Could you check a few things on this model? Use its own coordinates, in mm. A direction names the side the tool comes from. Round coordinates to 2 decimals unless told otherwise and drop trailing zeros. Write each loop counter-clockwise with the first axis right and the second up, starting at its lowest first coordinate (ties: lowest second). Pieces come first, ordered by that corner, then holes. Notation, with made-up numbers: (33, 73.5) -> (83, 73.5) arc R25 ccw to (83, 95.5) -> close; hole circle Ø4 at (-31, 27.5). An arc over 180 degrees is marked (long way). One line per question, with ' | ' between items. Start each with the question number.
1. Thinking about a two-plate mould opening in X: for faces 4 (the flat face through (12.7, 1.5, -4.1)), 5 (the flat face through (7, 0.8, -4)), 6 (the flat face through (9.064, 2.803, -3.514)), 7 (the flat face through (6, -1, -8)), which applies, released by +X, released by -X, zero draft, split by the parting line, or undercut?
2. Imagine slicing it at B-B, the plane z = -1. List the corners of the cut face in (x, y) for me.
3. If I drill on line 1 along Y through (x, z) = (11.5, -1); line 2 along Y through (x, z) = (8.25, -3.75); line 3 along Z through (x, y) = (7.25, -0.5), over which ranges is the centre line in solid material (lowest first)? Write a range as [from, to].
4. Imagine slicing it at A-A, the plane y = 0.5. List the corners of the cut face in (x, z) for me, and give its area (3 significant figures).
5. For faces 1 (the flat face through (4, 2.6, -4)), 2 (the cylindrical face through (5.811, 0.394, -5.413)), 3 (the flat face through (6, -1, -7)), which set-ups out of +Z, -Z, +X, -X, +Y, -Y let a thin tool reach every point of the face, with its end or its side?
6. For pin 1 Ø1 at (x, z) = (2.5, -6) entering from -Y; pin 2 Ø1 at (x, y) = (11, -1.5) entering from +Z; pin 3 Ø0.6 at (x, y) = (8, -1) entering from +Z; pin 4 Ø1.5 at (x, z) = (4, -3.5) entering from +Y, each with a flat end and sliding along its axis, tell me the tip position at first contact or that it passes through.
7. Imagine slicing it at D-D, the plane y = 2.05. List the corners of the cut face in (x, z) for me.
8. Imagine slicing it at C-C, the plane x = 5.5. List the corners of the cut face in (y, z) for me.
from build123d import *

# Parameters (mm, degrees)
SKETCH1_W               = 13
SKETCH1_H               = 8
BOSS_EXTRUDE1_DEPTH     = 3
CUT_EXTRUDE1_DEPTH      = 16.556349186
CUT_EXTRUDE1_DEPTH_BACK = 16.556349186
CUT_EXTRUDE2_DEPTH      = 16.556349186
CUT_EXTRUDE2_DEPTH_BACK = 16.556349186
SKETCH4_R               = 1.8
CUT_EXTRUDE3_DEPTH      = 0.8
SKETCH5_W               = 8
SKETCH5_H               = 1
BOSS_EXTRUDE2_DEPTH     = 2
FILLET1_R               = 4
SKETCH6_W               = 0.576923077
SKETCH6_H               = 3
CUT_EXTRUDE4_DEPTH      = 0.4


with BuildPart() as part:
    # Sketch1 → Boss-Extrude1 (new body)
    with BuildSketch(Plane(origin=(0, 0, 0), x_dir=(1, 0, 0), z_dir=(0, 1, 0))):
        with Locations((6.5, 4)):
            Rectangle(SKETCH1_W, SKETCH1_H)
    extrude(amount=BOSS_EXTRUDE1_DEPTH)

    # Sketch2 → Cut-Extrude1 (cut, two sides: drawn at the far end of the back side and taken through both)
    with BuildSketch(Plane.XY.offset(-CUT_EXTRUDE1_DEPTH_BACK)):
        Polygon((0, 0), (0.6, 3), (0, 3), align=None)
        Polygon((13, 0), (12.4, 3), (13, 3), align=None)
    extrude(amount=CUT_EXTRUDE1_DEPTH + CUT_EXTRUDE1_DEPTH_BACK, mode=Mode.SUBTRACT)

    # Sketch3 → Cut-Extrude2 (cut, two sides: drawn at the far end of the back side and taken through both)
    with BuildSketch(Plane(origin=(0, 0, 0), x_dir=(0, 0, -1), z_dir=(1, 0, 0)).offset(-CUT_EXTRUDE2_DEPTH_BACK)):
        Polygon((0, 0), (0.6, 3), (0, 3), align=None)
        Polygon((8, 3), (7.4, 3), (8, 0), align=None)
    extrude(amount=CUT_EXTRUDE2_DEPTH + CUT_EXTRUDE2_DEPTH_BACK, mode=Mode.SUBTRACT)

    # Sketch4 → Cut-Extrude3 (cut)
    with BuildSketch(Plane.XZ):
        with Locations(Location((6.50000125, -3.75, 0), (0, 0, 270))):
            Circle(SKETCH4_R)
    extrude(amount=-CUT_EXTRUDE3_DEPTH, mode=Mode.SUBTRACT)

    # Sketch5 → Boss-Extrude2 (add)
    with BuildSketch(Plane.XZ):
        with Locations((6.500011, -7.5)):
            Rectangle(SKETCH5_W, SKETCH5_H)
    extrude(amount=BOSS_EXTRUDE2_DEPTH)

    # Fillet1
    # the kernel refuses this fillet: 4 mm, written as the material it takes off along each edge
    with BuildSketch(Plane(origin=(10.500011, -2, -16.660254038), x_dir=(0, 1, 0), z_dir=(0, 0, 1)), Plane(origin=(2.500011, -2, 1.660254038), x_dir=(0, 1, 0), z_dir=(0, 0, -1))) as fillet1_piece_1:
        with BuildLine():
            CenterArc((4, 3.464101615), FILLET1_R, 180, 60)
            Line((0, 3.464101615), (-0.08, 3.464101615))
            Line((-0.08, 3.464101615), (-0.08, 0))
            Line((-0.08, 0), (0, -0.08))
            ThreePointArc((0, -0.08), (1, -0.08), (1.96, -0.069282032))
            Line((1.96, -0.069282032), (2, 0))
        make_face()
    extrude(amount=18.320508076, mode=Mode.SUBTRACT)

    # Sketch6 → Cut-Extrude4 (cut)
    with BuildSketch(Plane(origin=(0, 3, 0), x_dir=(1, 0, 0), z_dir=(0, 1, 0))):
        Polygon((3.219165588, 2.557267472), (2.50101655, 5.557267472), (3.092362704, 5.557267472), (3.558708858, 3.496570357), (4.052098281, 5.557267472), (4.839357896, 5.557267472), (5.327939627, 3.461714587), (5.793083858, 5.557267472), (6.385631934, 5.557267472), (5.68070405, 2.557267472), (4.966160781, 2.557267472), (4.443324242, 4.800055934), (3.906665588, 2.557267472), align=None)
        with Locations((6.981785781, 4.057267472)):
            Rectangle(SKETCH6_W, SKETCH6_H)
        Polygon((7.885631934, 2.557267472), (7.885631934, 5.557267472), (8.488396358, 5.557267472), (9.693324242, 3.584911703), (9.693324242, 5.557267472), (10.270247319, 5.557267472), (10.270247319, 2.557267472), (9.648853088, 2.557267472), (8.462555011, 4.498373241), (8.462555011, 2.557267472), align=None)
    extrude(amount=-CUT_EXTRUDE4_DEPTH, mode=Mode.SUBTRACT)


solid = part.part
Geometry results:
1) face 4: released by +X | face 5: undercut | face 6: undercut | face 7: zero draft
2) outline: (0, 0) -> (13, 0) -> (12.4, 3) -> (0.6, 3) -> close
3) line 1: y = [0, 3] | line 2: y = [0.8, 2.6] | line 3: z = [-8, -7]
4) outline: (0.1, -7.9) -> (12.9, -7.9) -> (12.9, -0.1) -> (0.1, -0.1) -> close; hole circle Ø3.6 at (6.5, -3.75) | area: 89.7 mm2
5) face 1: +Y | face 2: -Y | face 3: +Z, +X, -X, -Y
6) pin 1: stops at y = 0 | pin 2: passes through | pin 3: stops at z = -7 | pin 4: stops at y = 3
7) outline: (0.41, -7.59) -> (12.59, -7.59) -> (12.59, -0.41) -> (0.41, -0.41) -> close
8) outline: (-1.97, -8) -> (0, -8) -> (3, -7.4) -> (3, -4.24) -> (2.6, -4.24) -> (2.6, -2.56) -> (3, -2.56) -> (3, -0.6) -> (0, 0) -> (0, -2.25) -> (0.8, -2.25) -> (0.8, -5.25) -> (0, -5.25) -> (0, -7) -> (-1.97, -7) -> close
